Check sheet for the drawn part. Datum: minimum x, y, z corner. Units: mm. A direction names the side the tool comes from. Coordinates: 2 decimals unless noted, no trailing zeros. Order: outer loops, then holes, each group sorted by start corner. A loop starts at its lowest first (then second) coordinate and runs counter-clockwise, first axis right, second up. Notation, with made-up numbers: M 9.5,-7 L 67.5,-7 A27 ccw 67.5,18 Z; hole C 65.5,51 d8. An arc over 180 degrees is marked long. Answer in a Markdown table with one row per item. Add a question column.
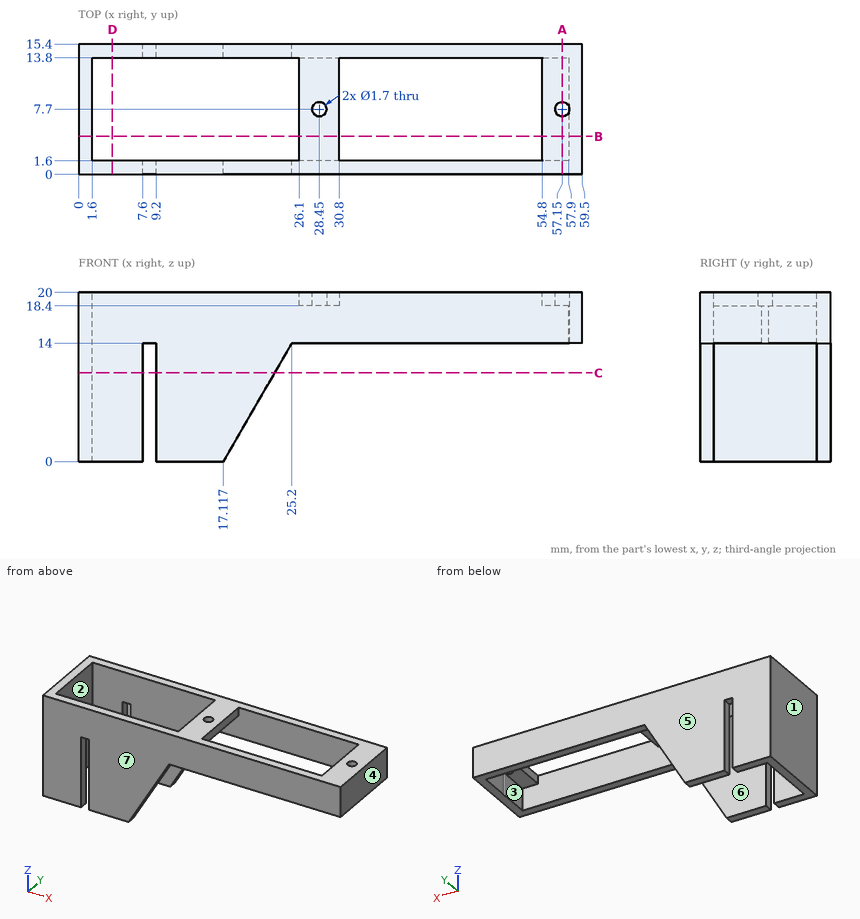
1. Section check B-B on y = 4.5. Enter the section's corners in (x, z).
2. Scan lines: line 1 (X direction, y = 7.7, z = 19.5); line 2 (Y direction, x = 15.5, z = 18); line 3 (X direction, y = 4.75, z = 18.75). Record each from-to range of solid material in increasing order.
3. Section check A-A on x = 57.15. Enter the section's corners in (y, z), then the cut area to 3 significant figures.
4. Set-up check for the marked faces 1, 2 and 3: record each of +Z, -Z, +X, -X, +Y, -Y from which the full face is reachable in a straight line by a thin tool's end or side.
5. Section check C-C on z = 10.5. Enter the section's corners in (x, y).
6. Section check D-D on x = 4. Enter the section's corners in (y, z).
7. Go/stop test with flat-tipped pins: pin 1 Ø1.3 at (y, z) = (14, 5) entering from +X; pin 2 Ø1.8 at (y, z) = (0.5, 7) entering from +X; pin 3 Ø5 at (x, y) = (28.5, 5) entering from -Z. Record where each tip stops, or that it passes through.
8. Release check for a two-part mould opening along Y. For the marked faces 4, 5, 6 and 7 record: released by +Y, released by -Y, zero draft, split by the parting line, or undercut.
Result sheet:
| question | item | result |
|---|---|---|
| 1 | outline | M 0,0 L 1.6,0 L 1.6,20 L 0,20 Z; M 26.1,18.4 L 30.8,18.4 L 30.8,20 L 26.1,20 Z; M 54.8,18.4 L 57.9,18.4 L 57.9,14 L 59.5,14 L 59.5,20 L 54.8,20 Z |
| 2 | line 1 | 0 to 1.6, 26.1 to 27.6, 29.3 to 30.8, 54.8 to 56.3, 58 to 59.5 |
| 2 | line 2 | 0 to 1.6, 13.8 to 15.4 |
| 2 | line 3 | 0 to 1.6, 26.1 to 30.8, 54.8 to 59.5 |
| 3 | outline | M 0,14 L 1.6,14 L 1.6,18.4 L 6.85,18.4 L 6.85,20 L 0,20 Z; M 8.55,18.4 L 13.8,18.4 L 13.8,14 L 15.4,14 L 15.4,20 L 8.55,20 Z |
| 3 | area | 36.0 mm^2 |
| 4 | face 1 | +Z, -Z, -X, +Y, -Y |
| 4 | face 2 | +Z, -Z |
| 4 | face 3 | -Z |
| 5 | outline | M 0,0 L 7.6,0 L 7.6,1.6 L 1.6,1.6 L 1.6,13.8 L 7.6,13.8 L 7.6,15.4 L 0,15.4 Z; M 9.2,0 L 23.18,0 L 23.18,1.6 L 9.2,1.6 Z; M 9.2,13.8 L 23.18,13.8 L 23.18,15.4 L 9.2,15.4 Z |
| 6 | outline | M 0,0 L 1.6,0 L 1.6,20 L 0,20 Z; M 13.8,0 L 15.4,0 L 15.4,20 L 13.8,20 Z |
| 7 | pin 1 | x = 20.38 |
| 7 | pin 2 | x = 21.68 |
| 7 | pin 3 | z = 18.4 |
| 8 | face 4 | zero draft |
| 8 | face 5 | released by +Y |
| 8 | face 6 | undercut |
| 8 | face 7 | released by -Y |
